Design review of the part built by this model. Coordinates are the model's own, in mm. A direction names the side the tool comes from. Give positions to 0.01 mm unless a question says otherwise; leave off trailing zeros. Loops run counter-clockwise (first coordinate to the right, second up) from the corner with the lowest first, then second, coordinate; pieces in that order, holes last. Notation, with made-up numbers: M 22,57.25 L 78,57.25 A27 cw 78,89.25 Z; hole C -30,48.5 d8. An arc over 180 degrees is marked long. Use a Markdown table: item, result. Add a question column.
(1) Add section B-B, the plane x = 0. Give the boundary of the cut face in (y, z), then the cut area to 3 significant figures.
(2) For probe 1 along X at (y, z) = (-205, -725); probe 2 along Y at (x, z) = (-51, -366.5); probe 3 along Z at (x, y) = (-32, -94), list the stretches that pass through material, from the lowest coordinate up.
(3) Draft analysis for pull direction X (two halves, no side actions). For faces 1 (the face through (150, -123, -688)), 2 (the face through (-277, -123, -815.008)), 3 (the face through (400, -123, -413)), state which applies: pulls with the +X half, pulls with the -X half, needs draft (parallel to the pull), parting line crosses it, or undercut.
(4) Add section C-C, the plane y = -90. Give the boundary of the cut face in (x, z), then the cut area to 3 significant figures.
(5) Add section A-A, the plane z = -605.5. Give the boundary of the cut face in (x, y), then the cut area to 3 significant figures.
(6) For faces 4 (the face through (-128.982, -348.6, 118.273)), 5 (the face through (-6, 0, -199)), 6 (the face through (-150, -123, -692)), list the 3-axis set-ups (+Z, -Z, +X, -X, +Y, -Y) from which the entire face can be reached by the end or side of a thin tool; tool diameter is ignored.
(7) Insertion check: pin 1 Ø12 at (x, z) = (-122.5, -476) entering from -Y; pin 2 Ø4 at (x, y) = (39, -91) entering from -Z; pin 3 Ø2 at (x, y) = (-144, -350) entering from -Z; pin 4 Ø1 at (x, z) = (-279, -276.5) entering from +Y. Each pin has a flat end and moves straight along its axis. Give the tip position at first contact, or say it passes through.
(8) Add section D-D, the plane z = -246.5. Give the boundary of the cut face in (x, y), then the cut area to 3 significant figures.
```python
from build123d import *

# Parameters (mm, degrees)
F1_DEPTH = 250
F2_R     = 175
F3_DEPTH = 200
F4_R     = 175
F5_DEPTH = 200


with BuildPart() as f1:
    # F0 (on Front) → F1 (new body)
    with BuildSketch(Plane.XZ):
        with BuildLine():
            Line((400, -815.00775), (400, 0))
            ThreePointArc((400, 0), (0, 400), (-400, 0))
            Line((-400, 0), (-400, -815.00775))
            Line((-400, -815.00775), (-150, -815.00775))
            Line((-150, -815.00775), (-150, -565.00775))
            Line((-150, -565.00775), (150, -565.00775))
            Line((150, -565.00775), (150, -815.00775))
            Line((150, -815.00775), (400, -815.00775))
        make_face()
    extrude(amount=F1_DEPTH)

    # F2 (on face) → F3 (join)
    with BuildSketch(Plane(origin=(0, 0, 0), x_dir=(-1, 0, 0), z_dir=(0, 1, 0))):
        Circle(F2_R)
    extrude(amount=-F3_DEPTH)

    # F4 (on face) → F5 (join)
    with BuildSketch(Plane.XZ.offset(250)):
        Circle(F4_R)
    extrude(amount=F5_DEPTH)


solid = f1.part
```
Established:
| question | item | result |
|---|---|---|
| 1 | outline | M -450,-175 L -250,-175 L -250,-565.01 L 0,-565.01 L 0,400 L -250,400 L -250,175 L -450,175 Z |
| 1 | area | 311,000 mm^2 |
| 2 | probe 1 | -400 to -150, 150 to 400 |
| 2 | probe 2 | -250 to 0 |
| 2 | probe 3 | -565.01 to 398.72 |
| 3 | face 1 | undercut |
| 3 | face 2 | needs draft |
| 3 | face 3 | pulls with the +X half |
| 4 | outline | M -400,-815.01 L -150,-815.01 L -150,-565.01 L 150,-565.01 L 150,-815.01 L 400,-815.01 L 400,0 A400 ccw -400,0 Z |
| 4 | area | 828,000 mm^2 |
| 5 | outline | M -400,-250 L -150,-250 L -150,0 L -400,0 Z; M 150,-250 L 400,-250 L 400,0 L 150,0 Z |
| 5 | area | 125,000 mm^2 |
| 6 | face 4 | -Y |
| 6 | face 5 | +Z, -Z, +X, -X, +Y |
| 6 | face 6 | -Z, +Y, -Y |
| 7 | pin 1 | y = -250 |
| 7 | pin 2 | z = -565.01 |
| 7 | pin 3 | z = -100.88 |
| 7 | pin 4 | y = 0 |
| 8 | outline | M -400,-250 L 400,-250 L 400,0 L -400,0 Z |
| 8 | area | 200,000 mm^2 |
